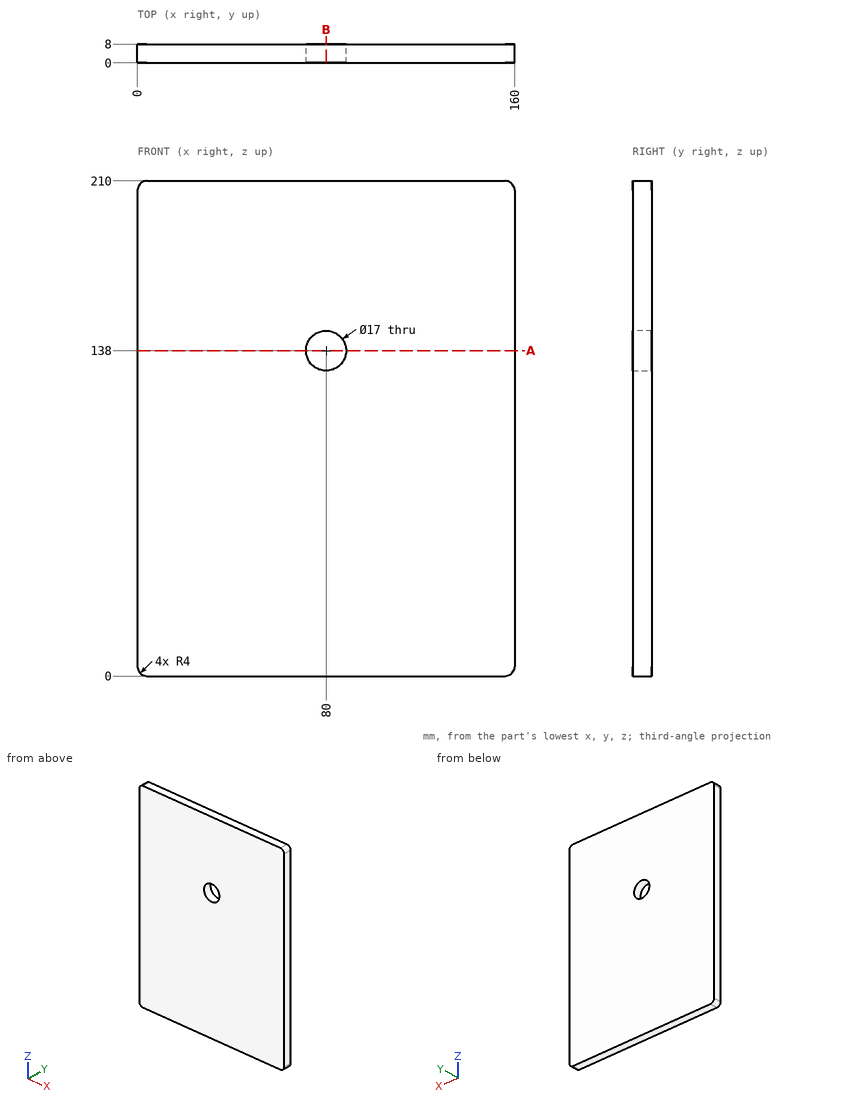
Check sheet for the drawn part. Datum: minimum x, y, z corner. Units: mm. Give positions to 0.01 mm unless a question says otherwise; leave off trailing zeros. Order: outer loops, then holes, each group sorted by start corner. A loop starts at its lowest first (then second) coordinate and runs counter-clockwise, first axis right, second up.
1. Sectioned sample at B-B (x = 80). Record the boundary of the cut face in (y, z), then the cut area to 3 significant figures.
Completed:
outline: (0, 0) - (8, 0) - (8, 129.5) - (0, 129.5) - close; (0, 146.5) - (8, 146.5) - (8, 210) - (0, 210) - close
area: 1,540 mm2
2. Scan lines: line 1 (X direction, y = 5.25, z = 138); line 2 (X direction, y = 4.75, z = 143). Record each from-to range of solid material in increasing order.
Completed:
line 1: x = 0 to 71.5, 88.5 to 160
line 2: x = 0 to 73.13, 86.87 to 160
3. Sectioned sample at A-A (z = 138). Record the boundary of the cut face in (x, y).
Completed:
outline: (0, 0) - (71.5, 0) - (71.5, 8) - (0, 8) - close; (88.5, 0) - (160, 0) - (160, 8) - (88.5, 8) - close
